CAD build for the part. Positions are in the model's coordinates, mm. A direction names the side the tool comes from. Coordinates: 2 decimals unless noted, no trailing zeros. Loops run counter-clockwise (first coordinate to the right, second up) from the corner with the lowest first, then second, coordinate; pieces in that order, holes last. Notation, with made-up numbers: (51, -16) - (90, -16) arc R18 cw to (90, -7) - close; hole circle Ø7 at (-26.5, -32.75). An arc over 180 degrees is marked (long way). Put each result on its own line as item: value.
```python
from build123d import *

# Parameters (mm, degrees)
F0_W     = 17.790004611
F0_H     = 67.7184760571
F0_R     = 11.8720680475
F1_DEPTH = 6


# Not quite as in the source:
# - a feature names something its author has since deleted; it is built from what else it names


with BuildPart() as f1:
    # F0 (on Front) → F1 (new body)
    with BuildSketch(Plane.XZ):
        with BuildLine():
            add(Edge.make_bspline(
                [(155.761959786, -128.1328057871), (178.7677402867, -122.1328057871), (178.7677402867, 81.1552154075), (178.761959786, 81.8671942129)],
                knots=[0, 0, 0, 0, 211.255769152, 211.255769152, 211.255769152, 211.255769152], degree=3))
            Line((178.761959786, 81.8671942129), (157.261959786, 81.8671942129))
            Line((157.261959786, 81.8671942129), (157.261959786, 76.8671942129))
            Line((157.261959786, 76.8671942129), (135.761959786, 76.8671942129))
            Line((135.761959786, 76.8671942129), (135.761959786, -108.1328057871))
            Line((135.761959786, -108.1328057871), (145.761959786, -108.1328057871))
            Line((145.761959786, -108.1328057871), (145.761959786, -128.1328057871))
            Line((145.761959786, -128.1328057871), (155.761959786, -128.1328057871))
        make_face()
        with Locations((151.5024825931, -66.7420731425)):
            Rectangle(F0_W, F0_H, mode=Mode.SUBTRACT)
        with Locations((155.7367742062, 29.270966208)):
            Circle(F0_R, mode=Mode.SUBTRACT)
    extrude(amount=F1_DEPTH)


solid = f1.part
```
Q1. Slice it at C-C, the plane y = -1. State how many separate pieces and enclosed holes the cut face has, then the cut area to 3 significant figures.
Determined:
separate pieces: 1
enclosed holes: 2
area: 6,070 mm2
Q2. Wall check: L1, parallel to Z at x = 156.5, y = -5.5; L2, parallel to Z at x = 157, y = -0.5; L3, parallel to Z at x = 140, y = -3.25. Give the ranges that are in metal, low to high. Write a range as from..to.
Determined:
L1: -127.87..-100.6, -32.88..17.42, 41.12..76.87
L2: -127.61..-100.6, -32.88..17.47, 41.08..76.87
L3: -108.13..76.87
Q3. Tool access for faces 1 (the flat face through (147, -3, 76.867)), 2 (the flat face through (160.397, -3, -67)), 3 (the flat face through (151, -3, -128.133)), 4 (the flat face through (141, -3, -108.133)): list every direction of +Z, -Z, +X, -X, +Y, -Y with a clear straight run to the whole face (end or side of a thin tool).
Determined:
face 1: +Z, -X, +Y, -Y
face 2: +Y, -Y
face 3: -Z, +X, -X, +Y, -Y
face 4: -Z, -X, +Y, -Y
Q4. Slice it at A-A, the plane x = 154. Give the cut face in (y, z), then the cut area to 3 significant figures.
Determined:
outline: (-6, -128.13) - (0, -128.13) - (0, -100.6) - (-6, -100.6) - close; (-6, -32.88) - (0, -32.88) - (0, 17.53) - (-6, 17.53) - close; (-6, 41.02) - (0, 41.02) - (0, 76.87) - (-6, 76.87) - close
area: 683 mm2
Q5. Slice it at B-B, the plane x = 139.5. Give the cut face in (y, z).
Determined:
outline: (-6, -108.13) - (0, -108.13) - (0, 76.87) - (-6, 76.87) - close
Q6. Pin check, flat tips, straight feed: pin 1 Ø3 at (x, y) = (141.5, -4) entering from -Z; pin 2 Ø1.8 at (x, y) = (148.5, -4) entering from +Z; pin 3 Ø2 at (x, z) = (159, -43.5) entering from -Y; pin 4 Ø1.8 at (y, z) = (-3, -52.5) entering from +X. Stop position of each tip, or through.
Determined:
pin 1: z = -108.13
pin 2: z = 76.87
pin 3: through
pin 4: x = 173.82
Q7. Mould opens along X. For faces 5 (the flat face through (157, 0, 2)), 6 (the flat face through (151, -3, -100.601)), 7 (the flat face through (157.262, -3, 79)) say: +X half, -X half, draft (parallel to the pull), parting line (faces both ways), or undercut.
Determined:
face 5: draft
face 6: undercut
face 7: -X half
